The drawing under review shows one solid part. Ordinate dimensions are in mm from its lowest x, y, z. A direction names the side the tool comes from. Round coordinates to 2 decimals unless told otherwise and drop trailing zeros. Order: outer loops, then holes, each group sorted by start corner. A loop starts at its lowest first (then second) coordinate and runs counter-clockwise, first axis right, second up. Notation, with made-up numbers: M 60,85 L 85,85 A22 ccw 85,119 Z; hole C -17,41 d10. An arc over 180 degrees is marked long. Answer as a JSON object with one key per item and string values. Group by question number.
1. To check wall thickness, follow probe 1 along X at (y, z) = (2, 20); probe 2 along X at (y, z) = (2.25, 2.5); probe 3 along X at (y, z) = (0.85, 2.5). State the ranges of each line that lie inside material, in increasing order. Write a range as [from, to].
2. Add section D-D on x = 2.5. State the section outline as (y, z) points, and give its area (3 significant figures).
3. Machinability: for the marked faces 1 and 2, which of the approach directions +Z, -Z, +X, -X, +Y, -Y give a long, thin tool a straight path to every point of the face, cutting with its end or side? Answer none if there is none.
4. Add section A-A on z = 20. State the section outline as (x, y) points.
5. Clearance check with flat-ended pins moving along their axes: P1, Ø2.5, axis at x = 22, y = 2, coming from the +Z side; P2, Ø3, axis at y = 6, z = 20.5, coming from the -X side; P3, Ø9, axis at x = 2, z = 18, coming from the +Y side; P4, Ø2.5, axis at x = 36, z = 2.5, coming from the +Y side. State where each tip first meets the part, or that it passes through.
6. Add section B-B on y = 1. State the section outline as (x, z) points, and give its area (3 significant figures).
7. Add section C-C on z = 26.5. State the section outline as (x, y) points.
8. Mouldability with a two-part tool opening along X and no side actions: class the marked faces 3, 4 and 5 as released by +X, released by -X, zero draft, split by the parting line, or undercut.
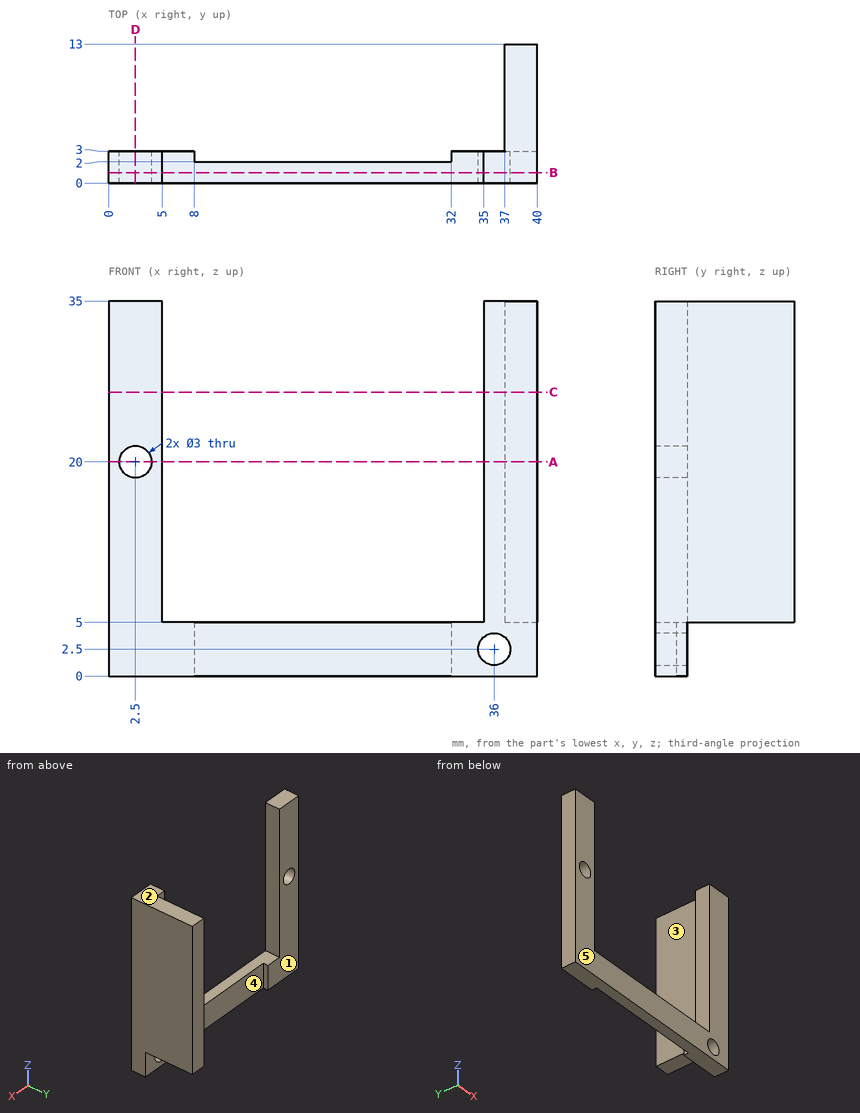
Recorded:
{
 "1": {"probe 1": "x = [0, 1], [4, 5], [35, 40]", "probe 2": "x = [0, 8], [32, 34.5], [37.5, 40]", "probe 3": "x = [0, 34.5], [37.5, 40]"},
 "2": {"outline": "M 0,0 L 3,0 L 3,18.5 L 0,18.5 Z; M 0,21.5 L 3,21.5 L 3,35 L 0,35 Z", "area": "96.0 mm²"},
 "3": {"face 1": "+Z, -Z, -X, +Y", "face 2": "+Z, +X, -X, +Y, -Y"},
 "4": {"outline": "M 0,0 L 1,0 L 1,3 L 0,3 Z; M 4,0 L 5,0 L 5,3 L 4,3 Z; M 35,0 L 40,0 L 40,13 L 37,13 L 37,3 L 35,3 Z"},
 "5": {"P1": "stops at z = 5", "P2": "stops at x = 37", "P3": "stops at y = 3", "P4": "passes through"},
 "6": {"outline": "M 0,0 L 40,0 L 40,35 L 35,35 L 35,5 L 5,5 L 5,35 L 0,35 Z; hole C 2.5,20 d3; hole C 36,2.5 d3", "area": "486 mm²"},
 "7": {"outline": "M 0,0 L 5,0 L 5,3 L 0,3 Z; M 35,0 L 40,0 L 40,13 L 37,13 L 37,3 L 35,3 Z"},
 "8": {"face 3": "released by -X", "face 4": "undercut", "face 5": "zero draft"}
}
